```python
from build123d import *

# Parameters (mm, degrees)
CROQUIS1_W              = 17
CROQUIS1_H              = 15
SALIENTE_EXTRUIR1_DEPTH = 32
VACIADO1_T              = -0.8
CORTAR_EXTRUIR1_DEPTH   = 32
CROQUIS3_W              = 5
CROQUIS3_H              = 15
SALIENTE_EXTRUIR2_DEPTH = 6.5
CROQUIS4_W              = 5
CROQUIS4_H              = 15
SALIENTE_EXTRUIR3_DEPTH = 6.5
CORTAR_EXTRUIR2_DEPTH   = 6.5
CROQUIS6_W              = 1.5
CROQUIS6_H              = 5.2
CORTAR_EXTRUIR3_DEPTH   = 10
CROQUIS7_W              = 8
CROQUIS7_H              = 13
SALIENTE_EXTRUIR4_DEPTH = 5
CROQUIS8_W              = 8
CROQUIS8_H              = 13
SALIENTE_EXTRUIR5_DEPTH = 5
CROQUIS9_W              = 5
CROQUIS9_H              = 8
SALIENTE_EXTRUIR6_DEPTH = 45
CROQUIS10_W             = 5
CROQUIS10_H             = 5
SALIENTE_EXTRUIR7_DEPTH = 15
CROQUIS11_W             = 23
CROQUIS11_H             = 5
SALIENTE_EXTRUIR8_DEPTH = 11.5
CROQUIS12_W             = 23
CROQUIS12_H             = 5
SALIENTE_EXTRUIR9_DEPTH = 11.5


with BuildPart() as part:
    # Croquis1 → Saliente-Extruir1 (new body)
    with BuildSketch(Plane.XY):
        Rectangle(CROQUIS1_W, CROQUIS1_H)
    extrude(amount=SALIENTE_EXTRUIR1_DEPTH)

    # Vaciado1
    vaciado1_openings = [part.faces().sort_by_distance(p)[0] for p in [
        (0, 7.5, 16),
    ]]
    offset(amount=VACIADO1_T, openings=vaciado1_openings, kind=Kind.INTERSECTION)

    # Croquis2 → Cortar-Extruir1 (cut)
    with BuildSketch(Plane.XY.offset(32)):
        with BuildLine():
            Line((-6.5, 0), (-6.5, 7.5))
            Line((-6.5, 7.5), (6.5, 7.5))
            Line((6.5, 7.5), (6.5, 0))
            ThreePointArc((6.5, 0), (0, -6.5), (-6.5, 0))
        make_face()
    extrude(amount=-CORTAR_EXTRUIR1_DEPTH, mode=Mode.SUBTRACT)

    # Croquis3 → Saliente-Extruir2 (add)
    with BuildSketch(Plane(origin=(8.5, 0, 0), x_dir=(0, 0, -1), z_dir=(1, 0, 0))):
        with Locations((-29.5, 0)):
            Rectangle(CROQUIS3_W, CROQUIS3_H)
    extrude(amount=SALIENTE_EXTRUIR2_DEPTH)

    # Croquis4 → Saliente-Extruir3 (add)
    with BuildSketch(Plane.ZY.offset(8.5)):
        with Locations((29.5, 0)):
            Rectangle(CROQUIS4_W, CROQUIS4_H)
    extrude(amount=SALIENTE_EXTRUIR3_DEPTH)

    # Croquis5 → Cortar-Extruir2 (cut)
    with BuildSketch(Plane.XY.offset(32)):
        with BuildLine():
            Line((-13.5, 2.6), (-13.5, -2.6))
            ThreePointArc((-13.5, -2.6), (-12.4, -3.7), (-11.3, -2.6))
            Line((-11.3, -2.6), (-11.3, 2.6))
            ThreePointArc((-11.3, 2.6), (-12.4, 3.7), (-13.5, 2.6))
        make_face()
        with BuildLine():
            Line((11.3, 2.6), (11.3, -2.6))
            ThreePointArc((11.3, -2.6), (12.4, -3.7), (13.5, -2.6))
            Line((13.5, -2.6), (13.5, 2.6))
            ThreePointArc((13.5, 2.6), (12.4, 3.7), (11.3, 2.6))
        make_face()
    extrude(amount=-CORTAR_EXTRUIR2_DEPTH, mode=Mode.SUBTRACT)

    # Croquis6 → Cortar-Extruir3 (cut)
    with BuildSketch(Plane.XY.offset(32)):
        with Locations((-14.25, 0)):
            Rectangle(CROQUIS6_W, CROQUIS6_H)
        with Locations((14.25, 0)):
            Rectangle(CROQUIS6_W, CROQUIS6_H)
    extrude(amount=-CORTAR_EXTRUIR3_DEPTH, mode=Mode.SUBTRACT)

    # Croquis7 → Saliente-Extruir4 (add)
    with BuildSketch(Plane(origin=(8.5, 0, 0), x_dir=(0, 0, -1), z_dir=(1, 0, 0))):
        with Locations((-5, 0)):
            Rectangle(CROQUIS7_W, CROQUIS7_H)
    extrude(amount=SALIENTE_EXTRUIR4_DEPTH)

    # Croquis8 → Saliente-Extruir5 (add)
    with BuildSketch(Plane.ZY.offset(8.5)):
        with Locations((5, 0)):
            Rectangle(CROQUIS8_W, CROQUIS8_H)
    extrude(amount=SALIENTE_EXTRUIR5_DEPTH)

    # Croquis9 → Saliente-Extruir6 (add)
    with BuildSketch(Plane(origin=(0, 6.5, 0), x_dir=(1, 0, 0), z_dir=(0, 1, 0))):
        with Locations((-11, -5)):
            Rectangle(CROQUIS9_W, CROQUIS9_H)
        with Locations((11, -5)):
            Rectangle(CROQUIS9_W, CROQUIS9_H)
    extrude(amount=SALIENTE_EXTRUIR6_DEPTH)

    # Croquis10 → Saliente-Extruir7 (add)
    with BuildSketch(Plane.XY.offset(9)):
        with Locations((-11, 49)):
            Rectangle(CROQUIS10_W, CROQUIS10_H)
        with Locations((11, 49)):
            Rectangle(CROQUIS10_W, CROQUIS10_H)
    extrude(amount=SALIENTE_EXTRUIR7_DEPTH)

    # Croquis11 → Saliente-Extruir8 (add)
    with BuildSketch(Plane(origin=(-8.5, 0, 0), x_dir=(0, 0, -1), z_dir=(1, 0, 0))):
        with Locations((-12.5, 49)):
            Rectangle(CROQUIS11_W, CROQUIS11_H)
    extrude(amount=SALIENTE_EXTRUIR8_DEPTH)

    # Croquis12 → Saliente-Extruir9 (add)
    with BuildSketch(Plane.ZY.offset(-8.5)):
        with Locations((12.5, 49)):
            Rectangle(CROQUIS12_W, CROQUIS12_H)
    extrude(amount=SALIENTE_EXTRUIR9_DEPTH)


solid = part.part
```
For this review, take the finished solid that the model builds, in its own axes (mm). A direction names the side the tool comes from. Round coordinates to 2 decimals unless told otherwise and drop trailing zeros. Write each loop counter-clockwise with the first axis right and the second up, starting at its lowest first coordinate (ties: lowest second). Pieces come first, ordered by that corner, then holes. Notation, with made-up numbers: (11, 13) - (66, 13) arc R23 ccw to (66, 25) - close; hole circle Ø8 at (63.25, 17). An arc over 180 degrees is marked (long way). Answer as a JSON object with one key per item and string values.
1. To check wall thickness, follow line 1 along Y through (x, z) = (5.25, 9.5); line 2 along X through (y, z) = (0.5, 5); line 3 along Y through (x, z) = (-8, 25.5). State the ranges of each line that lie inside material, in increasing order.
Response values:
{"line 1": "y = -7.5 to -6.7, 46.5 to 51.5", "line 2": "x = -13.5 to -7.7, 7.7 to 13.5", "line 3": "y = -7.5 to 7.5"}
2. For pin 1 Ø0.9 at (y, z) = (3.5, 0.5) entering from -X; pin 2 Ø10 at (y, z) = (3.5, 10) entering from +X; pin 3 Ø2.5 at (x, y) = (11, 22.5) entering from +Z; pin 4 Ø10 at (x, y) = (-0.5, -0.5) entering from +Z, all flat-tipped, find the tip position at first contact; note any pin that passes through.
Response values:
{"pin 1": "stops at x = -8.5", "pin 2": "stops at x = 13.5", "pin 3": "stops at z = 9", "pin 4": "passes through"}
3. We need section B-B on z = 22. Give the boundary of the cut face in (x, y).
Response values:
{"outline": "(-13.5, 46.5) - (13.5, 46.5) - (13.5, 51.5) - (-13.5, 51.5) - close; (-8.5, -7.5) - (8.5, -7.5) - (8.5, 7.5) - (7.7, 7.5) - (7.7, -6.7) - (-7.7, -6.7) - (-7.7, 7.5) - (-8.5, 7.5) - close"}
4. We need section C-C on y = 18. Give the boundary of the cut face in (x, z).
Response values:
{"outline": "(-13.5, 1) - (-8.5, 1) - (-8.5, 9) - (-13.5, 9) - close; (8.5, 1) - (13.5, 1) - (13.5, 9) - (8.5, 9) - close"}
5. We need section D-D on z = 28. Give the boundary of the cut face in (x, y).
Response values:
{"outline": "(-15, -7.5) - (15, -7.5) - (15, -2.6) - (13.5, -2.6) arc R1.1 cw to (11.3, -2.6) - (11.3, 2.6) arc R1.1 cw to (13.5, 2.6) - (15, 2.6) - (15, 7.5) - (7.7, 7.5) - (7.7, -6.7) - (-7.7, -6.7) - (-7.7, 7.5) - (-15, 7.5) - (-15, 2.6) - (-13.5, 2.6) arc R1.1 cw to (-11.3, 2.6) - (-11.3, -2.6) arc R1.1 cw to (-13.5, -2.6) - (-15, -2.6) - close"}
6. We need section A-A on x = 2.5. Give the boundary of the cut face in (y, z).
Response values:
{"outline": "(-7.5, 0) - (-6, 0) - (-6, 0.8) - (-6.7, 0.8) - (-6.7, 31.2) - (-6, 31.2) - (-6, 32) - (-7.5, 32) - close; (46.5, 1) - (51.5, 1) - (51.5, 24) - (46.5, 24) - close"}
7. Draft analysis for pull direction X (two halves, no side actions). For faces 4 (the face through (-12.4, 3.7, 29.5)), 5 (the face through (9, 22, 1)), 6 (the face through (-13.5, 29, 7)), state which applies: +X half, -X half, draft (parallel to the pull), parting line (faces both ways), or undercut.
Response values:
{"face 4": "undercut", "face 5": "draft", "face 6": "-X half"}
8. Tool access review of faces 1 (the face through (12.4, -3.7, 29.5)), 2 (the face through (-11, 0, 27)), 3 (the face through (14, -2.6, 30)): name each direction out of +Z, -Z, +X, -X, +Y, -Y from which nothing blocks a thin tool from reaching the whole face with its end or side.
Response values:
{"face 1": "+Z", "face 2": "-X, +Y, -Y", "face 3": "+Z, -Z, +X"}
